Read the model definition and answer for the solid it produces. Units are mm, in the model's axes. A direction names the side the tool comes from. Give positions to 0.01 mm unless a question says otherwise; leave off trailing zeros. Order: outer loops, then holes, each group sorted by start corner. A loop starts at its lowest first (then second) coordinate and runs counter-clockwise, first axis right, second up. Notation, with made-up numbers: (89.5, 80) - (131.5, 80) arc R18 cw to (131.5, 114) - close; hole circle Ø2 at (40, 18). An arc over 180 degrees is marked (long way). Return JSON: item names as keys, results as strings.
Autodesk Inventor part; units mm, degrees
ref_plane "YZ Plane" through (0, 0, 0) normal (1, 0, 0) x (0, 1, 0)
ref_plane "XZ Plane" through (0, 0, 0) normal (0, 1, 0) x (-1, 0, 0)
ref_plane "XY Plane" through (0, 0, 0) normal (0, 0, 1) x (1, 0, 0)
sketch "Sketch1" plane through (0, 0, 0) normal (0, 0, 1) x (1, 0, 0)
  arc A0 (0, -3) -> (3, 0) centre (0, 0) ccw
  line L0 (3, 12) -> (3, 0)
  arc A1 (3, 12) -> (0, 15) centre (0, 12) ccw
  line L1 (-34, 15) -> (0, 15)
  arc A2 (-34, 15) -> (-37, 12) centre (-34, 12) ccw
  line L2 (-37, 0) -> (-37, 12)
  arc A3 (-37, 0) -> (-34, -3) centre (-34, 0) ccw
  line L3 (0, -3) -> (-34, -3)
  arc A4 (-32.9749, 5.5) -> (-28, 1) centre (-28, 6) ccw
  arc A5 (-28, 10) -> (-32.9749, 5.5) centre (-28, 5) ccw
  line L4 (-6, 10) -> (-28, 10)
  arc A6 (-1.0251, 5.5) -> (-6, 10) centre (-6, 5) ccw
  arc A7 (-6, 1) -> (-1.0251, 5.5) centre (-6, 6) ccw
  line L5 (-28, 1) -> (-6, 1)
  line L6 (-37.75, 0) -> (-37.75, 12)
  line L7 (3.75, 12) -> (3.75, 0)
  line L8 (0, 0) -> (0.75, 0)
  line L9 (0, 12) -> (0.75, 12)
  line L10 (-34, 12) -> (-34.75, 12)
  line L11 (-34, 0) -> (-34.75, 0)
  arc A8 (-37.75, 0) -> (-34.75, -3) centre (-34.75, 0) ccw
  line L12 (-34.75, 0) -> (-34.75, -3) construction
  line L13 (-34.75, 0) -> (-31.75, 0) construction
  arc A9 (0.75, -3) -> (3.75, 0) centre (0.75, 0) ccw
  arc A10 (3.75, 12) -> (0.75, 15) centre (0.75, 12) ccw
  arc A11 (-34.75, 15) -> (-37.75, 12) centre (-34.75, 12) ccw
  line L14 (-34.75, 12) -> (-34.75, 15) construction
  line L15 (-34.75, 12) -> (-37.75, 12) construction
  line L16 (-34, -3) -> (-34.75, -3)
  line L17 (-34, 15) -> (-34.75, 15)
  line L18 (0, 15) -> (0.75, 15)
  line L19 (0, -3) -> (0.75, -3)
  line L20 (-34, 15) -> (0, 15)
  line L21 (-34, -3) -> (0, -3)
  line L22 (-38.25, 12) -> (-38.25, 0)
  arc A12 (-38.25, 0) -> (-34.75, -3.5) centre (-34.75, 0) ccw
  line L23 (-34.75, -3.5) -> (-34, -3.5)
  line L24 (-34, -3.5) -> (0, -3.5)
  line L25 (0, -3.5) -> (0.75, -3.5)
  arc A13 (0.75, -3.5) -> (4.25, 0) centre (0.75, 0) ccw
  line L26 (4.25, 0) -> (4.25, 12)
  arc A14 (4.25, 12) -> (0.75, 15.5) centre (0.75, 12) ccw
  line L27 (0.75, 15.5) -> (0, 15.5)
  line L28 (0, 15.5) -> (-34, 15.5)
  line L29 (-34, 15.5) -> (-34.75, 15.5)
  arc A15 (-34.75, 15.5) -> (-38.25, 12) centre (-34.75, 12) ccw
  line L30 (-41.75, 12) -> (-41.75, 0)
  arc A16 (-41.75, 0) -> (-34.75, -7) centre (-34.75, 0) ccw
  line L31 (-34.75, -7) -> (-34, -7)
  line L32 (-34, -7) -> (0, -7)
  line L33 (0, -7) -> (0.75, -7)
  arc A17 (0.75, -7) -> (7.75, 0) centre (0.75, 0) ccw
  line L34 (7.75, 0) -> (7.75, 12)
  arc A18 (7.75, 12) -> (0.75, 19) centre (0.75, 12) ccw
  line L35 (0.75, 19) -> (0, 19)
  line L36 (0, 19) -> (-34, 19)
  line L37 (-34, 19) -> (-34.75, 19)
  arc A19 (-34.75, 19) -> (-41.75, 12) centre (-34.75, 12) ccw
  point P0 (0, 0)
  dimension "d1" = 40
  dimension "d4" = 0.75
  dimension "d5" = 0.75
  dimension "d6" = 0.75
  dimension "d7" = 0.75
  dimension "d8" = 0.75
  dimension "d9" = 90
  dimension "d10" = 90
  dimension "d11" = 0.5
  dimension "d12" = 3.5
extrude "Extrusion1" add sketch "Sketch1" against normal blind 35 contours A19 L37 L36 L35 A18 L34 A17 L33 L32 L31 A16 L30
sketch "Sketch2" plane through (0, 0, 0) normal (0, 0, 1) x (1, 0, 0)
  line L0 (-41.75, 12) -> (-41.75, 0)
  line L1 (7.75, 0) -> (7.75, 12)
  line L2 (7.75, 6) -> (17.75, 6)
  line L3 (-41.75, 6) -> (-51.75, 6)
  line L4 (-41.75, 8.5) -> (-51.75, 8.5)
  line L5 (-41.75, 3.5) -> (-51.75, 3.5)
  line L6 (7.75, 8.5) -> (17.75, 8.5)
  line L7 (7.75, 3.5) -> (17.75, 3.5)
  line L8 (17.75, 8.5) -> (7.75, 8.5)
  line L9 (7.75, 8.5) -> (7.75, 3.5)
  line L10 (7.75, 3.5) -> (17.75, 3.5)
  line L11 (17.75, 3.5) -> (17.75, 8.5)
  line L12 (-51.75, 8.5) -> (-41.75, 8.5)
  line L13 (-41.75, 8.5) -> (-41.75, 3.5)
  line L14 (-41.75, 3.5) -> (-51.75, 3.5)
  line L15 (-51.75, 3.5) -> (-51.75, 8.5)
  point P0 (0, 0)
  dimension "d15" = 10
  dimension "d16" = 10
  dimension "d17" = 2.5
  dimension "d18" = 2.5
  dimension "d19" = 2.5
  dimension "d20" = 2.5
extrude "Extrusion2" add sketch "Sketch2" against normal up to surface (35 mm away)
sketch "Sketch3" plane through (7.75, 3.5, 0) normal (0, -1, 0) x (1, 0, 0)
  line L0 (10, -35) -> (0, -35)
  line L1 (10, 0) -> (10, -35)
  line L2 (0, 0) -> (10, 0)
  line L3 (0, -35) -> (0, 0)
  line L4 (-49.5, -35) -> (-59.5, -35)
  line L5 (-49.5, 0) -> (-49.5, -35)
  line L6 (-59.5, 0) -> (-49.5, 0)
  line L7 (-59.5, 0) -> (-59.5, -35)
  circle A0 centre (5, -5) radius 5
  circle A1 centre (5, -30) radius 5
  circle A2 centre (-54.5, -5) radius 5
  circle A3 centre (-54.5, -30) radius 5
  circle A4 centre (-54.5, -5) radius 1.5
  circle A5 centre (-54.5, -30) radius 1.5
  circle A6 centre (5, -5) radius 1.5
  circle A7 centre (5, -30) radius 1.5
  point P0 (-7.75, 0)
  dimension "d23" = 3
  dimension "d24" = 3
  dimension "d25" = 3
  dimension "d26" = 3
extrude "Extrusion3" cut sketch "Sketch3" against normal blind 10 contours A4 | A5 | A6 | A7
sketch "Sketch4" plane through (-34.75, -7, 0) normal (0, -1, 0) x (1, 0, 0)
  line L0 (0, 0) -> (35.5, 0)
  line L1 (17.75, 0) -> (17.75, -26)
  line L2 (17.75, -26) -> (17.75, -31)
  circle A0 centre (17.75, -28.5) radius 2.5
  circle A1 centre (17.75, -28.5) radius 1.4
  point P0 (34.75, 0)
  dimension "d29" = 26
  dimension "d30" = 5
  dimension "d31" = 2.8
extrude "Extrusion4" cut sketch "Sketch4" against normal blind 10 contours A1 L2 | L2 A1
equation "\"d21\" = d18"
properties part number "camHolder_3DPrint"
Q1. A cutting plane is placed at A-A (y = 4.75). Write down the section's boundary in (x, z), and give its area (3 significant figures).
Values:
{"outline": "(-51.75, -35) - (-38.25, -35) - (-38.25, 0) - (-51.75, 0) - close; (4.25, -35) - (17.75, -35) - (17.75, 0) - (4.25, 0) - close; hole circle Ø3 at (-46.75, -30); hole circle Ø3 at (-46.75, -5); hole circle Ø3 at (12.75, -30); hole circle Ø3 at (12.75, -5)", "area": "917 mm²"}
Q2. Determine the mould class of faces 1 (the cylindrical face through (12.555, 5.965, -3.513)), 2 (the cylindrical face through (-47.86, 5.96, -28.99)), 3 (the flat face through (-17, -4, 0)), 4 (the flat face through (-17, 15.5, -17)) for opening direction Z: released by +Z, released by -Z, zero draft, split by the parting line, or undercut.
Values:
{"face 1": "undercut", "face 2": "undercut", "face 3": "released by +Z", "face 4": "zero draft"}
Q3. A cutting plane is placed at B-B (x = -46.75). Write down the section's boundary in (y, z), and give its area (3 significant figures).
Values:
{"outline": "(3.5, -35) - (8.5, -35) - (8.5, -31.5) - (3.5, -31.5) - close; (3.5, -28.5) - (8.5, -28.5) - (8.5, -6.5) - (3.5, -6.5) - close; (3.5, -3.5) - (8.5, -3.5) - (8.5, 0) - (3.5, 0) - close", "area": "145 mm²"}
Q4. A cutting plane is placed at C-C (z = -12). Write down the section's boundary in (x, y).
Values:
{"outline": "(-51.75, 3.5) - (-41.75, 3.5) - (-41.75, 0) arc R7 ccw to (-34.75, -7) - (0.75, -7) arc R7 ccw to (7.75, 0) - (7.75, 3.5) - (17.75, 3.5) - (17.75, 8.5) - (7.75, 8.5) - (7.75, 12) arc R7 ccw to (0.75, 19) - (-34.75, 19) arc R7 ccw to (-41.75, 12) - (-41.75, 8.5) - (-51.75, 8.5) - close; hole (-38.25, 0) arc R3.5 ccw to (-34.75, -3.5) - (0.75, -3.5) arc R3.5 ccw to (4.25, 0) - (4.25, 12) arc R3.5 ccw to (0.75, 15.5) - (-34.75, 15.5) arc R3.5 ccw to (-38.25, 12) - close"}
Q5. A cutting plane is placed at D-D (x = -0.5). Write down the section's boundary in (y, z), and give its area (3 significant figures).
Values:
{"outline": "(-7, -35) - (-3.5, -35) - (-3.5, 0) - (-7, 0) - close; (15.5, -35) - (19, -35) - (19, 0) - (15.5, 0) - close", "area": "245 mm²"}
Q6. Consider L1, parallel to Z at x = -46.75, y = 4.9; L2, parallel to Y at x = -14.5, z = -10; L3, parallel to Y at x = -48, z = -19.5. Determine where each line is inside the solid, lowest interval first.
Values:
{"L1": "z = -35 to -31.5, -28.5 to -6.5, -3.5 to 0", "L2": "y = -7 to -3.5, 15.5 to 19", "L3": "y = 3.5 to 8.5"}
Q7. Given pin 1 (1 mm diameter, centred on y = 11, z = -12.5, fed in from -X); pin 2 (8 mm diameter, centred on x = 12.5, z = -13.5, fed in from +Y); pin 3 (6 mm diameter, centred on y = 13, z = -17, fed in from +X); pin 4 (2.5 mm diameter, centred on x = 12.75, z = -30, fed in from -Y), each flat-ended and moving along its own axis, determine where each tip first touches the part or whether it passes through.
Values:
{"pin 1": "stops at x = -41.75", "pin 2": "stops at y = 8.5", "pin 3": "stops at x = 7.75", "pin 4": "passes through"}
Q8. For faces 5 (the flat face through (13, 8.5, -17)), 6 (the flat face through (-41.75, 10, -17)), 7 (the cylindrical face through (3.3, 14.4, -17.3)), 8 (the flat face through (7.75, 2, -17)), determine the directions among +Z, -Z, +X, -X, +Y, -Y from which every point of the face is accessible in a straight line to the end or side of a thin tool.
Values:
{"face 5": "+Z, -Z, +X, +Y", "face 6": "+Z, -Z, -X, +Y", "face 7": "+Z, -Z", "face 8": "+Z, -Z, +X, -Y"}
